Verification items for the finished model (mm, model axes). Face numbers are marked on the shaded views. Coordinates: 2 decimals unless noted, no trailing zeros. Write each loop counter-clockwise with the first axis right and the second up, starting at its lowest first coordinate (ties: lowest second). Pieces come first, ordered by that corner, then holes. Notation, with made-up numbers: M -37.5,68.25 L 13.5,68.25 A10 ccw 13.5,82.25 Z; hole C 75,56 d8. An arc over 180 degrees is marked long. One line per item, written item: value.
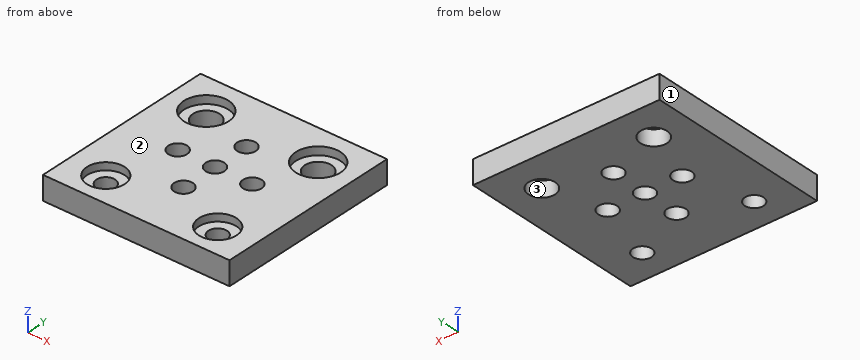
Autodesk Inventor part; units mm, degrees
ref_plane "Work Plane1" through (0, -18.83, 0) normal (-1, 0, 0) x (0, 0, 1)
ref_plane "YZ Plane" through (0, 0, 0) normal (1, 0, 0) x (0, 1, 0)
ref_plane "XZ Plane" through (0, 0, 0) normal (0, 1, 0) x (-1, 0, 0)
sketch "Sketch1" plane through (0, 0, 0) normal (0, 0, 1) x (1, 0, 0)
  line L0 (-25, -25) -> (25, -25)
  line L1 (25, -25) -> (25, 25)
  line L2 (25, 25) -> (-25, 25)
  line L3 (-25, 25) -> (-25, -25)
  line L4 (-25, -25) -> (25, 25) construction
  line L5 (25, -25) -> (-25, 25) construction
  point P0 (0, 0)
  dimension "Width" = 50
  dimension "Height" = 50
extrude "Extrusion1" add sketch "Sketch1" along normal blind 6.35
sketch "Sketch2" plane through (0, 0, 6.35) normal (0, 0, 1) x (1, 0, 0)
  line L0 (-25, -25) -> (25, -25)
  line L1 (25, -25) -> (25, 25)
  line L2 (25, 25) -> (-25, 25)
  line L3 (-25, 25) -> (-25, -25)
  line L4 (0, 25) -> (0, -25) construction
  line L5 (-25, 0) -> (25, 0) construction
  point P0 (0, 0)
  point P1 (0, 0)
  point P2 (-10, 0)
  point P3 (0, 10)
  point P4 (0, -10)
  point P5 (10, 0)
  dimension "d4" = 10
  dimension "d5" = 10
  dimension "d6" = 10
  dimension "d7" = 10
hole "Hole1" at (0, 0, 6.35) at (-10, 0, 6.35) at (0, 10, 6.35) at (0, -10, 6.35) at (10, 0, 6.35) direction (0, 0, -1) diameter 5.02 end through all
sketch "Sketch3" plane through (0, 0, 6.35) normal (0, 0, 1) x (1, 0, 0)
  line L0 (-25, -25) -> (25, -25)
  line L1 (25, -25) -> (25, 25)
  line L2 (25, 25) -> (-25, 25)
  line L3 (-25, 25) -> (-25, -25)
  line L4 (0, 25) -> (0, -25) construction
  line L5 (25, 0) -> (-25, 0) construction
  line L6 (15, 25) -> (15, -25) construction
  line L7 (-25, -15) -> (25, -15) construction
  point P0 (15, 15)
  point P1 (-15, 15)
  dimension "d15" = 15
  dimension "d16" = 15
hole "Hole2" at (-15, 15, 6.35) at (15, 15, 6.35) direction (0, 0, -1) diameter 7.14 end through all counterbore diameter 12 counterbore depth 2.18
sketch "Sketch6" plane through (0, 0, 6.35) normal (0, 0, 1) x (1, 0, 0)
  circle A0 centre (-15, 15) radius 6
  circle A1 centre (15, 15) radius 6
  circle A2 centre (0, -10) radius 2.51
  circle A3 centre (-10, 0) radius 2.51
  circle A4 centre (0, 0) radius 2.51
  circle A5 centre (0, 10) radius 2.51
  circle A6 centre (10, 0) radius 2.51
  line L0 (-25, -25) -> (25, -25)
  line L1 (25, -25) -> (25, 25)
  line L2 (25, 25) -> (-25, 25)
  line L3 (-25, 25) -> (-25, -25)
sketch "Sketch7" plane through (0, 0, 6.35) normal (0, 0, 1) x (1, 0, 0)
  circle A0 centre (-15, 15) radius 6
  circle A1 centre (15, 15) radius 6
  line L0 (-25, -25) -> (25, -25)
  line L1 (25, -25) -> (25, 25)
  line L2 (-25, 25) -> (-25, -25)
  line L3 (15, 15) -> (15, -25) construction
  line L4 (25, -16.9) -> (-25, -16.9) construction
  line L5 (-15, 15) -> (-15, -16.9) construction
  point P0 (15, -16.9)
  dimension "d35" = 31.9
hole "Hole3" at (-15, -16.9, 6.35) at (15, -16.9, 6.35) direction (0, 0, -1) diameter 5 end through all counterbore diameter 10.1 counterbore depth 2
sketch "Sketch4" plane through (0, 0, 6.35) normal (0, 0, 1) x (1, 0, 0)
  line L0 (25, -18.83) -> (25, 18.83)
  line L1 (-25, 18.83) -> (-25, -18.83)
  line L2 (-25, 0) -> (25, 0) construction
  line L3 (-22.25, 3.35) -> (-19.75, 3.35)
  line L4 (-19.75, 3.35) -> (-19.75, -3.35)
  line L5 (-19.75, -3.35) -> (-22.25, -3.35)
  line L6 (-22.25, -3.35) -> (-22.25, 3.35)
  line L7 (-22.25, 3.35) -> (-19.75, -3.35) construction
  line L8 (-19.75, 3.35) -> (-22.25, -3.35) construction
  point P0 (-21, 0)
  dimension "d25" = 2.5
  dimension "d27" = 5.25
  dimension "d28" = 6.7
sketch "Sketch5" plane through (-25, -18.83, 0) normal (-1, 0, 0) x (0, 0, 1)
  line L0 (6.35, 37.66) -> (6.35, 0)
  line L1 (0, 15.48) -> (0, 22.18)
  line L2 (6.35, 22.18) -> (0, 22.18)
  line L3 (6.35, 15.48) -> (0, 15.48)
  line L4 (6.35, 22.18) -> (4.17, 22.18)
  line L5 (4.17, 22.18) -> (4.17, 15.48)
  line L6 (4.17, 15.48) -> (6.35, 15.48)
  line L7 (6.35, 15.48) -> (6.35, 22.18)
  point P0 (0, 18.83)
  dimension "d31" = 2.18
properties part number "Micro V Plate" material "Aluminum 6061"
Item 1: Draft check along X on the marked faces 1, 2 and 3. Enter one of: released by +X, released by -X, zero draft, split by the parting line, or undercut.
The answers:
face 1: released by -X
face 2: zero draft
face 3: undercut
Item 2: Cross-section at C-C, the plane z = 2.5. Give the number of separate pieces and of enclosed holes in the cut face, and give its area (3 significant figures).
The answers:
separate pieces: 1
enclosed holes: 9
area: 2,280 mm²
Item 3: Cross-section at A-A, the plane y = -16.9. Enter the section's corners in (x, z), and give its area (3 significant figures).
The answers:
outline: M -25,0 L -17.5,0 L -17.5,4.35 L -20.05,4.35 L -20.05,6.35 L -25,6.35 Z; M -12.5,0 L 12.5,0 L 12.5,4.35 L 9.95,4.35 L 9.95,6.35 L -9.95,6.35 L -9.95,4.35 L -12.5,4.35 Z; M 17.5,0 L 25,0 L 25,6.35 L 20.05,6.35 L 20.05,4.35 L 17.5,4.35 Z
area: 234 mm²
Item 4: Scan lines: line 1 (X direction, y = -16.9, z = 5.25); line 2 (Y direction, x = 0, z = 2.25); line 3 (X direction, y = 15, z = 5.1). Record each from-to range of solid material in increasing order.
The answers:
line 1: x = -25 to -20.05, -9.95 to 9.95, 20.05 to 25
line 2: y = -25 to -12.51, -7.49 to -2.51, 2.51 to 7.49, 12.51 to 25
line 3: x = -25 to -21, -9 to 9, 21 to 25
Item 5: Go/stop test with flat-tipped pins: P1, Ø8, axis at x = -15, y = -16.9, coming from the +Z side; P2, Ø6, axis at x = 15.5, y = 17, coming from the +Z side. Record where each tip stops, or that it passes through.
The answers:
P1: stops at z = 4.35
P2: stops at z = 4.17
Item 6: Cross-section at B-B, the plane x = 15. Enter the section's corners in (y, z).
The answers:
outline: M -25,0 L -19.4,0 L -19.4,4.35 L -21.95,4.35 L -21.95,6.35 L -25,6.35 Z; M -14.4,0 L 11.43,0 L 11.43,4.17 L 9,4.17 L 9,6.35 L -11.85,6.35 L -11.85,4.35 L -14.4,4.35 Z; M 18.57,0 L 25,0 L 25,6.35 L 21,6.35 L 21,4.17 L 18.57,4.17 Z
Item 7: Cross-section at D-D, the plane y = 0. Enter the section's corners in (x, z), and give its area (3 significant figures).
The answers:
outline: M -25,0 L -12.51,0 L -12.51,6.35 L -25,6.35 Z; M -7.49,0 L -2.51,0 L -2.51,6.35 L -7.49,6.35 Z; M 2.51,0 L 7.49,0 L 7.49,6.35 L 2.51,6.35 Z; M 12.51,0 L 25,0 L 25,6.35 L 12.51,6.35 Z
area: 222 mm²
